Read the model definition and answer for the solid it produces. Units are mm, in the model's axes. Face numbers are marked on the shaded views. A direction names the side the tool comes from. Coordinates: 2 decimals unless noted, no trailing zeros. Write each loop counter-clockwise with the first axis right and the second up, starting at its lowest first coordinate (ties: lowest second). Pieces come first, ordered by that corner, then holes. Notation, with made-up numbers: (70.25, 74) -> (77.25, 74) arc R29 ccw to (77.25, 111) -> close; hole circle Ø7 at (-26, 60). An arc over 180 degrees is marked (long way). Write item = value, one per line. Start each with the question number.
1) Section A-A (y = 0) is taken. Determine the outline of the cut face in (x, z).
2) A tool of negligible diameter and unlimited length cuts with its end or side. For the marked faces 1 and 2, from which of +Z, -Z, +X, -X, +Y, -Y can it reach the whole face along a straight path? Write none if from no direction.
3) Flat-ended cylindrical pins translate along their axes: pin 1 Ø8 at (x, y) = (0.5, -3) entering from +Z; pin 2 Ø5 at (x, y) = (-5, 4) entering from +Z. Find the tip coordinate at first contact, or state that the pin passes through.
4) For a pull along X with two mould halves and no side action, classify the marked faces 3, 4, 5 and 6 as released by +X, released by -X, zero draft, split by the parting line, or undercut.
5) Find the intervals of material crossed by line 1 along Z through (x, y) = (0, 3.25); line 2 along Z through (x, y) = (-5.25, 6), in increasing order. Write a range as from..to.
6) Section C-C (x = -0.25) is taken. Determine the outline of the cut face in (y, z), plus the area to 3 significant figures.
7) Section B-B (z = 59) is taken. Determine the outline of the cut face in (x, y), plus the area to 3 significant figures.
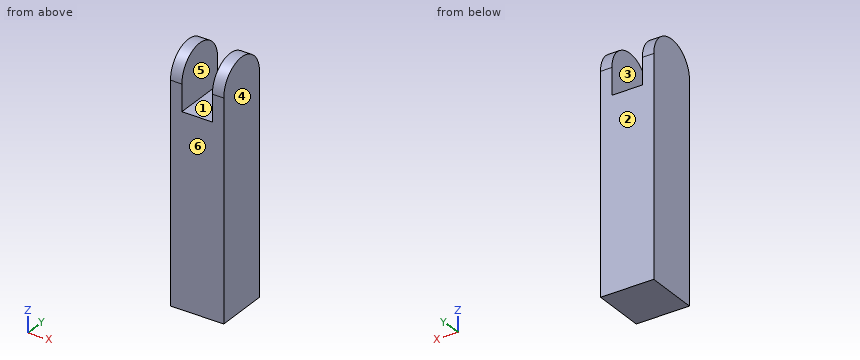
from build123d import *

# Parameters (mm, degrees)
SKETCH_1_W          = 14
SKETCH_1_H          = 14
EXTRUDE_1_DEPTH     = 64
CUT_EXTRUDE_1_DEPTH = 64
SKETCH_3_W          = 8
SKETCH_3_H          = 14
CUT_EXTRUDE_2_DEPTH = 15


with BuildPart() as part:
    # 草图1 → 凸台-拉伸1 (new body)
    with BuildSketch(Plane.XY):
        Rectangle(SKETCH_1_W, SKETCH_1_H)
    extrude(amount=EXTRUDE_1_DEPTH)

    # 草图2 → 切除-拉伸1 (cut)
    with BuildSketch(Plane(origin=(7, 0, 0), x_dir=(0, 0, -1), z_dir=(1, 0, 0))):
        with BuildLine():
            Line((-57, 7), (-68.546767236, 7))
            Line((-68.546767236, 7), (-68.546767236, -7))
            Line((-68.546767236, -7), (-57, -7))
            ThreePointArc((-57, -7), (-64, 0), (-57, 7))
        make_face()
    extrude(amount=-CUT_EXTRUDE_1_DEPTH, mode=Mode.SUBTRACT)

    # 草图3 → 切除-拉伸2 (cut, through all)
    with BuildSketch(Plane(origin=(0, 7, 0), x_dir=(1, 0, 0), z_dir=(0, 1, 0))):
        with Locations((0, -57)):
            Rectangle(SKETCH_3_W, SKETCH_3_H)
    extrude(amount=-CUT_EXTRUDE_2_DEPTH, mode=Mode.SUBTRACT)


solid = part.part
Answer key:
q1.outline = (-7, 0) -> (7, 0) -> (7, 64) -> (4, 64) -> (4, 50) -> (-4, 50) -> (-4, 64) -> (-7, 64) -> close
q2.face_1 = +Z, +Y, -Y
q2.face_2 = +Z, -Z, +X, -X, +Y
q3.pin_1 = 63.92
q3.pin_2 = 63.84
q4.face_3 = undercut
q4.face_4 = released by +X
q4.face_5 = undercut
q4.face_6 = zero draft
q5.line_1 = 0..50
q5.line_2 = 0..60.61
q6.outline = (-7, 0) -> (7, 0) -> (7, 50) -> (-7, 50) -> close
q6.area = 700 mm^2
q7.outline = (-7, -6.71) -> (-4, -6.71) -> (-4, 6.71) -> (-7, 6.71) -> close; (4, -6.71) -> (7, -6.71) -> (7, 6.71) -> (4, 6.71) -> close
q7.area = 80.5 mm^2
